```python
from build123d import *

# Parameters (mm, degrees)
SKETCH1_W           = 80
SKETCH1_H           = 80
BOSS_EXTRUDE1_DEPTH = 4
SKETCH2_R           = 1.6
CUT_EXTRUDE1_DEPTH  = 114.207773585
LPATTERN1_COUNT     = 6
LPATTERN1_PITCH     = 10
SKETCH3_W           = 80
SKETCH3_H           = 3
BOSS_EXTRUDE2_DEPTH = 18
SKETCH4_R           = 1.6
CUT_EXTRUDE2_DEPTH  = 113.485554628
LPATTERN2_COUNT     = 2
LPATTERN2_PITCH     = 5
FILLET1_R           = 6
FILLET2_R           = 6


with BuildPart() as part:
    # Sketch1 → Boss-Extrude1 (new body)
    with BuildSketch(Plane.XY):
        with Locations((40, 40)):
            Rectangle(SKETCH1_W, SKETCH1_H)
    extrude(amount=BOSS_EXTRUDE1_DEPTH)

    # Sketch2 → Cut-Extrude1 (cut, through all)
    with BuildSketch(Plane.XY.offset(4)):
        with Locations((10, 70)):
            Circle(SKETCH2_R)
        with Locations((25, 70)):
            Circle(SKETCH2_R)
        with Locations((40, 70)):
            Circle(SKETCH2_R)
        with Locations((55, 70)):
            Circle(SKETCH2_R)
        with Locations((70, 70)):
            Circle(SKETCH2_R)
    cut_extrude1 = extrude(amount=-CUT_EXTRUDE1_DEPTH, mode=Mode.SUBTRACT)

    # LPattern1: Cut-Extrude1 ×6
    with Locations(*[(0, -i * LPATTERN1_PITCH, 0) for i in range(1, LPATTERN1_COUNT)]):
        add(cut_extrude1, mode=Mode.SUBTRACT)

    # Sketch3 → Boss-Extrude2 (add)
    with BuildSketch(Plane(origin=(0, 0, 0), x_dir=(-1, 0, 0), z_dir=(0, 0, -1))):
        with Locations((-40, 1.5)):
            Rectangle(SKETCH3_W, SKETCH3_H)
    extrude(amount=BOSS_EXTRUDE2_DEPTH)

    # Sketch4 → Cut-Extrude2 (cut, through all)
    with BuildSketch(Plane(origin=(0, 3, 0), x_dir=(1, 0, 0), z_dir=(0, 1, 0))):
        with Locations(Location((70, 15, 0), (0, 0, 270))):
            Circle(SKETCH4_R)
        with Locations(Location((55, 15, 0), (0, 0, 270))):
            Circle(SKETCH4_R)
        with Locations(Location((40, 15, 0), (0, 0, 270))):
            Circle(SKETCH4_R)
        with Locations(Location((25, 15, 0), (0, 0, 270))):
            Circle(SKETCH4_R)
        with Locations(Location((10, 15, 0), (0, 0, 270))):
            Circle(SKETCH4_R)
    cut_extrude2 = extrude(amount=-CUT_EXTRUDE2_DEPTH, mode=Mode.SUBTRACT)

    # LPattern2: Cut-Extrude2 ×2
    with Locations(*[(0, 0, i * LPATTERN2_PITCH) for i in range(1, LPATTERN2_COUNT)]):
        add(cut_extrude2, mode=Mode.SUBTRACT)

    # Fillet1
    fillet1_edges = [part.edges().sort_by_distance(p)[0] for p in [
        (40, 3, 0),
    ]]
    fillet(fillet1_edges, radius=FILLET1_R)

    # Fillet2
    fillet2_edges = [part.edges().sort_by_distance(p)[0] for p in [
        (80, 1.5, -18),
        (0, 1.5, -18),
        (0, 80, 2),
        (80, 80, 2),
    ]]
    fillet(fillet2_edges, radius=FILLET2_R)


solid = part.part
```
Check sheet for the modelled part. Datum: model origin and axes. Units: mm. Round coordinates to 2 decimals unless told otherwise and drop trailing zeros. Order: outer loops, then holes, each group sorted by start corner. A loop starts at its lowest first (then second) coordinate and runs counter-clockwise, first axis right, second up. Notation, with made-up numbers: (44.25, -25) - (51.25, -25) arc R16 cw to (51.25, -9) - close; hole circle Ø3 at (0, 2). An arc over 180 degrees is marked (long way). Answer as CSV lines item,"result". Start each with the question number.
1) Depth check by flat-ended pin: pin 1 (1.9 mm diameter, centred on x = 70, y = 20, fed in from +Z); pin 2 (8 mm diameter, centred on x = 9, z = -5.5, fed in from +Y); pin 3 (4 mm diameter, centred on x = 55, y = 20, fed in from -Z). Enter the tip coordinate at first touch or a pass-through.
2) Draft check along Y on faces 1 (the face through (71.48, 39.39, 2.03)), 2 (the face through (9.03, 1.52, -11.27)), 3 (the face through (40, 80, 2)). Enter one of: +Y half, -Y half, draft (parallel to the pull), parting line (faces both ways), or undercut.
3) Section check B-B (x = 64). Record the cut outline in (y, z), then the cut area to 3 significant figures.
4) Section check A-A (y = 50). Record the cut outline in (x, z), then the cut area to 3 significant figures.
5) Scan lines: probe 1 along Z at (x, y) = (74.5, 40); probe 2 along Y at (x, z) = (6, -14); probe 3 along X at (y, z) = (0.85, -15). Record each from-to range of solid material in increasing order.
6) Section check C-C (z = 2.75). Give the number of separate pieces and of enclosed holes in the cut face, then the cut area to 3 significant figures.
Determined:
1,pin 1,"through"
1,pin 2,"y = 5.03"
1,pin 3,"z = 0"
2,face 1,"undercut"
2,face 2,"draft"
2,face 3,"+Y half"
3,outline,"(0, -18) - (3, -18) - (3, -6) arc R6 cw to (9, 0) - (80, 0) - (80, 4) - (0, 4) - close"
3,area,"382 mm^2"
4,outline,"(0, 0) - (8.4, 0) - (8.4, 4) - (0, 4) - close; (11.6, 0) - (23.4, 0) - (23.4, 4) - (11.6, 4) - close; (26.6, 0) - (38.4, 0) - (38.4, 4) - (26.6, 4) - close; (41.6, 0) - (53.4, 0) - (53.4, 4) - (41.6, 4) - close; (56.6, 0) - (68.4, 0) - (68.4, 4) - (56.6, 4) - close; (71.6, 0) - (80, 0) - (80, 4) - (71.6, 4) - close"
4,area,"256 mm^2"
5,probe 1,"0 to 4"
5,probe 2,"0 to 3"
5,probe 3,"0.8 to 8.4, 11.6 to 23.4, 26.6 to 38.4, 41.6 to 53.4, 56.6 to 68.4, 71.6 to 79.2"
6,separate pieces,"1"
6,enclosed holes,"30"
6,area,"6,140 mm^2"
